Source: CAD feature listing. Evaluate the final solid. Frame: model axes, mm. Face numbers are marked on the shaded views. A direction names the side the tool comes from. Round coordinates to 2 decimals unless told otherwise and drop trailing zeros. Write each loop counter-clockwise with the first axis right and the second up, starting at its lowest first coordinate (ties: lowest second). Pieces come first, ordered by that corner, then holes. Notation, with made-up numbers: M -15.75,62.5 L 3.25,62.5 A20 ccw 3.25,101.5 Z; hole C 25,7 d10. An arc over 180 degrees is marked long. Answer in a Markdown table with one row per item.
from build123d import *

# Parameters (mm, degrees)
F0_W      = 5.08
F0_H      = 254
F1_DEPTH  = 76.2
F2_W      = 76.2
F2_H      = 228.6
F3_DEPTH  = 2.54
F4_W      = 254
F4_H      = 228.6
F5_DEPTH  = 12.7
F6_W      = 254
F6_H      = 228.6
F7_DEPTH  = 203.2
F8_W      = 244.1982476321
F8_H      = 219.8302176212
F9_DEPTH  = 203.2
F10_W     = 203.2
F10_H     = 101.6
F11_DEPTH = 25.4
F12_W     = 76.2
F12_H     = 177.8
F13_DEPTH = 25.4


with BuildPart() as f1:
    # F0 (on Top) → F1 (new body)
    with BuildSketch(Plane.XY):
        with Locations((78.74, -50.8)):
            Rectangle(F0_W, F0_H)
    extrude(amount=F1_DEPTH)

    # F2 (on Top) → F3 (join)
    with BuildSketch(Plane.XY):
        with Locations((38.1, -38.1)):
            Rectangle(F2_W, F2_H)
    extrude(amount=F3_DEPTH)

    # F4 (on Top) → F5 (join)
    with BuildSketch(Plane.XY):
        with Locations((-127, -38.1)):
            Rectangle(F4_W, F4_H)
    extrude(amount=F5_DEPTH)

    # F6 (on face) → F7 (join)
    with BuildSketch(Plane.XY.offset(12.7)):
        with Locations((-127, -38.1)):
            Rectangle(F6_W, F6_H)
    extrude(amount=F7_DEPTH)

    # F8 (on face) → F9 (cut)
    with BuildSketch(Plane.XY.offset(215.9)):
        with Locations((-126.820876184, -37.4048911894)):
            Rectangle(F8_W, F8_H)
    extrude(amount=-F9_DEPTH, mode=Mode.SUBTRACT)

    # F10 (on face) → F11 (cut)
    with BuildSketch(Plane.YZ):
        with Locations((-38.1, 139.7)):
            Rectangle(F10_W, F10_H)
    extrude(amount=-F11_DEPTH, mode=Mode.SUBTRACT)

    # F12 (on face) → F13 (cut)
    with BuildSketch(Plane.XZ.offset(152.4)):
        with Locations((-209.5483732462, 101.6)):
            Rectangle(F12_W, F12_H)
    extrude(amount=-F13_DEPTH, mode=Mode.SUBTRACT)


solid = f1.part
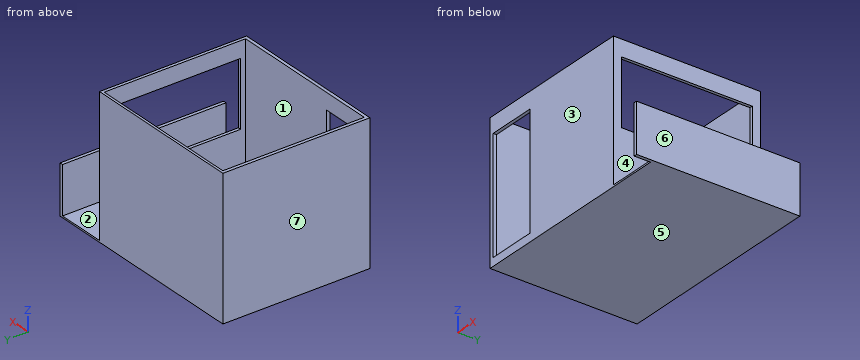
Q1. Section A-A (x = -220). Return loops of the section in (y, z), and give its area (3 significant figures).
Solutions:
| item | result |
|---|---|
| outline | M -152.4,0 L 76.2,0 L 76.2,215.9 L 72.51,215.9 L 72.51,12.7 L -152.4,12.7 Z; M -152.4,190.5 L -147.32,190.5 L -147.32,215.9 L -152.4,215.9 Z |
| area | 3,780 mm2 |
Q2. Section D-D (x = -131). Return loops of the section in (y, z), and give its area (3 significant figures).
Solutions:
| item | result |
|---|---|
| outline | M -152.4,0 L 76.2,0 L 76.2,215.9 L 72.51,215.9 L 72.51,12.7 L -147.32,12.7 L -147.32,215.9 L -152.4,215.9 Z |
| area | 4,690 mm2 |
Q3. Material intervals for probe 1 along X at (y, z) = (-60, 47.5); probe 2 along Y at (x, z) = (-74, 206.5); probe 3 along X at (y, z) = (5, 192), sorted ascending.
Solutions:
| item | result |
|---|---|
| probe 1 | x = -254 to -248.92, -4.72 to 0, 76.2 to 81.28 |
| probe 2 | y = -152.4 to -147.32, 72.51 to 76.2 |
| probe 3 | x = -254 to -248.92, -4.72 to 0 |
Q4. Section B-B (z = 23). Return loops of the section in (x, y).
Solutions:
| item | result |
|---|---|
| outline | M -254,-152.4 L -247.65,-152.4 L -247.65,-147.32 L -248.92,-147.32 L -248.92,72.51 L -4.72,72.51 L -4.72,-147.32 L -171.45,-147.32 L -171.45,-152.4 L 0,-152.4 L 0,76.2 L -254,76.2 Z; M 76.2,-177.8 L 81.28,-177.8 L 81.28,76.2 L 76.2,76.2 Z |
Q5. Pull-direction query (X, two-part tool) for the marked faces 4, 5, 6 and 7; classes: pulls with the +X half, pulls with the -X half, needs draft (parallel to the pull), parting line crosses it, or undercut.
Solutions:
| item | result |
|---|---|
| face 4 | undercut |
| face 5 | needs draft |
| face 6 | pulls with the +X half |
| face 7 | pulls with the -X half |
Q6. Access query for the marked faces 1, 2 and 3. Directions: +Z, -Z, +X, -X, +Y, -Y. A direction counts if a zero-diameter tool reaches every point of the face in a straight line with its end or side. Return the directions, or none.
Solutions:
| item | result |
|---|---|
| face 1 | +Z |
| face 2 | +Z, +Y, -Y |
| face 3 | +Z, -Z, -X, -Y |
Q7. Section C-C (y = 2). Return loops of the section in (x, z).
Solutions:
| item | result |
|---|---|
| outline | M -254,0 L 81.28,0 L 81.28,76.2 L 76.2,76.2 L 76.2,2.54 L 0,2.54 L 0,88.9 L -4.72,88.9 L -4.72,12.7 L -248.92,12.7 L -248.92,215.9 L -254,215.9 Z; M -4.72,190.5 L 0,190.5 L 0,215.9 L -4.72,215.9 Z |
Q8. Contact query for flat-ended pins moving along their axis: pin 1 Ø12 at (y, z) = (31, 191.5) entering from +X; pin 2 Ø1.4 at (x, z) = (-3.5, 153) entering from -Y; pin 3 Ø2.5 at (x, y) = (79.5, -112) entering from +Z. Output: stop coordinate, or through.
Solutions:
| item | result |
|---|---|
| pin 1 | stops at x = 0 |
| pin 2 | stops at y = -152.4 |
| pin 3 | stops at z = 76.2 |
